Could you check a few things on this model? Use its own coordinates, in mm. A direction names the side the tool comes from. Round coordinates to 2 decimals unless told otherwise and drop trailing zeros. Write each loop counter-clockwise with the first axis right and the second up, starting at its lowest first coordinate (ties: lowest second). Pieces come first, ordered by that corner, then holes. Notation, with made-up numbers: (-39, -27.75) -> (-9, -27.75) arc R25 ccw to (-9, -3.75) -> close; hole circle Ø8 at (49.25, -8). An arc over 180 degrees is marked (long way). Answer in a Markdown table with one row per item. Add a question column.
```python
from build123d import *

# Parameters (mm, degrees)
SKETCH2_R                        = 0.762
CHAMFER1_SIZE                    = 0.508
FILLET1_R                        = 0.254
F_10_32_TAPPED_HOLE1_D           = 4.0386
F_10_32_TAPPED_HOLE1_DEPTH       = 10.3124
F_10_32_TAPPED_HOLE1_CSINK_D     = 4.826
F_10_32_TAPPED_HOLE1_CSINK_ANGLE = 90
F_10_32_TAPPED_HOLE1_TIP         = 1.213317848


with BuildPart() as part:
    # Sketch1 → Revolve1 (revolve)
    with BuildSketch(Plane.XY, mode=Mode.PRIVATE) as revolve1_sk:
        Polygon((12.7, 0), (6.35, 0), (6.35, -6.35), (0, -6.35), (0, 29.21), (12.7, 7.212954744), align=None)
    revolve(revolve1_sk.sketch.rotate(Axis((0, 35.289344262, 0), (0, -1, 0)), 90), axis=Axis((0, 35.289344262, 0), (0, -1, 0)))  # turned: the seam where the file's is

    # Sketch2 → Cut-Revolve1 (revolve, cut)
    with BuildSketch(Plane.XY, mode=Mode.PRIVATE) as cut_revolve1_sk:
        with Locations((6.858, -0.508)):
            Circle(SKETCH2_R)
    revolve(cut_revolve1_sk.sketch.rotate(Axis((0, 0, 0), (0, -1, 0)), 90), axis=Axis((0, 0, 0), (0, -1, 0)), mode=Mode.SUBTRACT)  # turned: the seam where the file's is

    # Chamfer1
    chamfer1_edges = [part.edges().sort_by_distance(p)[0] for p in [
        (0, -6.35, -6.35),
    ]]
    chamfer(chamfer1_edges, length=CHAMFER1_SIZE)

    # Fillet1
    fillet1_edges = [part.edges().sort_by_distance(p)[0] for p in [
        (0, 0, -12.7),
    ]]
    fillet(fillet1_edges, radius=FILLET1_R)

    # 10-32 Tapped Hole1
    with Locations(Plane.XZ.offset(6.35)):
        with Locations((0, 0)):
            CounterSinkHole(F_10_32_TAPPED_HOLE1_D / 2, F_10_32_TAPPED_HOLE1_CSINK_D / 2, depth=F_10_32_TAPPED_HOLE1_DEPTH, counter_sink_angle=F_10_32_TAPPED_HOLE1_CSINK_ANGLE)
            with Locations((0, 0, -(F_10_32_TAPPED_HOLE1_DEPTH + F_10_32_TAPPED_HOLE1_TIP / 2))):  # 118° drill point
                Cone(0, F_10_32_TAPPED_HOLE1_D / 2, F_10_32_TAPPED_HOLE1_TIP, mode=Mode.SUBTRACT)


solid = part.part
```
(1) Suppose I cut it at C-C, the plane y = 18. Please give me the cut outline in (x, z), then the cut area to 3 significant figures.
(2) For P1, Ø3, axis at x = -3.5, y = 21.5, coming from the +Z side; P2, Ø10, axis at x = 9, z = 8.5, coming from the -Y side; P3, Ø4, axis at x = 3.5, z = 5, coming from the +Y side, each with a flat end and sliding along its axis, tell me the tip position at first contact or that it passes through.
(3) On a 3-axis mill with a long thin cutter (end or side, diameter ignored), from which of +Z, -Z, +X, -X, +Y, -Y can I reach the whole of each face in a straight line? I mean faces 1 (the face through (3.86, -3.49, -5.04)), 2 (the face through (3, -6.35, 0)). Say none if no direction works.
(4) Suppose I cut it at B-B, the plane y = 14. Please give me the cut outline in (x, z), then the cut area to 3 significant figures.
(5) If we mould it in two halves opening along Z, with no side actions, what happens to faces 3 (the face through (5.4, 0, 5.4)), 4 (the face through (-1.926, -0.928, 0.607)), 5 (the face through (-1.5, 20.5, 4.8))? For each: pulls with the +Z half, pulls with the -Z half, needs draft (parallel to the pull), parting line crosses it, or undercut.
(6) Suppose I cut it at A-A, the plane y = 2.5. Please give me the cut outline in (x, z), then the cut area to 3 significant figures.
(7) I need wall thicknesses on L1, parallel to X at y = -2.5, z = 0; L2, parallel to X at y = 1.25, z = 0; L3, parallel to Z at x = -4.25, y = 12.5. Which ranges of each line are inside material? Lowest first, please.
Response:
| question | item | result |
|---|---|---|
| 1 | outline | circle Ø12.94 at (0, 0) |
| 1 | area | 132 mm² |
| 2 | P1 | z = 4.44 |
| 2 | P2 | y = 0 |
| 2 | P3 | y = 22.1 |
| 3 | face 1 | -Y |
| 3 | face 2 | +Z, -Z, +X, -X, -Y |
| 4 | outline | circle Ø17.56 at (0, 0) |
| 4 | area | 242 mm² |
| 5 | face 3 | needs draft |
| 5 | face 4 | undercut |
| 5 | face 5 | parting line crosses it |
| 6 | outline | circle Ø25.4 at (0, 0); hole circle Ø4.04 at (0, 0) |
| 6 | area | 494 mm² |
| 7 | L1 | -6.35 to -2.02, 2.02 to 6.35 |
| 7 | L2 | -12.7 to -2.02, 2.02 to 12.7 |
| 7 | L3 | -8.66 to 8.66 |
